Source: CAD feature listing. Evaluate the final solid. Frame: model axes, mm. A direction names the side the tool comes from. Coordinates: 2 decimals unless noted, no trailing zeros. Loops run counter-clockwise (first coordinate to the right, second up) from the corner with the lowest first, then second, coordinate; pieces in that order, holes last. Notation, with made-up numbers: M -36,48.5 L 22,48.5 A30 ccw 22,76.5 Z; hole C 38.5,43.25 d11. An arc over 180 degrees is marked long. One line per question, with ' | ' between items. Start each with the question number.
1. Access query for faces 4 (the cylindrical face through (18.28, 39.51, -28.67)), 5 (the cylindrical face through (0, 2, 41)). Directions: +Z, -Z, +X, -X, +Y, -Y. A direction counts if a zero-diameter tool reaches every point of the face in a straight line with its end or side. Return the directions, or none.
2. Section query D-D, the plane z = 38.75. Output: boundary loops of the cut face in (x, y).
3. Section query C-C, the plane x = 38.75. Output: boundary loops of the cut face in (y, z), and give its area (3 significant figures).
4. Ray query, probe 1 along X at (y, z) = (2.5, 0); probe 2 along Y at (x, z) = (-18.5, -33); probe 3 along X at (y, z) = (2.95, 38.75). Return the intervals inside material, ascending.
5. Section query B-B, the plane z = 0. Output: boundary loops of the cut face in (x, y), and give its area (3 significant figures).
6. Section query A-A, the plane x = 0. Output: boundary loops of the cut face in (y, z), and give its area (3 significant figures).
7. Mould query, pull axis X, two halves, no side actions, for faces 1 (the cylindrical face through (0.099, 2.465, -36.502)), 2 (the flat face through (-1, 0, -1)), 3 (the cylindrical face through (-33.727, 2.465, 25.861)). Classes: pulls with the +X half, pulls with the -X half, needs draft (parallel to the pull), parting line crosses it, or undercut.
8. Pin query (flat end, axial travel): P1, Ø4, axis at x = 23, z = 34, coming from the +Y side; P2, Ø1.5, axis at x = -7, y = 48.5, coming from the +Z side; P3, Ø2, axis at y = 17, z = -21.5, coming from the -X side. Return the tip coordinate at first contact, or that it passes through.
```python
from build123d import *

# Parameters (mm, degrees)
ESQUISSE1_R        = 42.5
BOSS_EXTRU_2_DEPTH = 5
D_GAGEMENT_M42_D   = 4.5
ESQUISSE12_R       = 34
BOSS_EXTRU_3_DEPTH = 70


with BuildPart() as part:
    # Esquisse1 → Boss.-Extru.2 (new body)
    with BuildSketch(Plane(origin=(0, 0, 0), x_dir=(1, 0, 0), z_dir=(0, 1, 0))):
        Circle(ESQUISSE1_R)
    extrude(amount=BOSS_EXTRU_2_DEPTH)

    # Dégagement M42 (through all)
    with Locations(Plane(origin=(0, 5, -38.75), x_dir=(0, 0, 1), z_dir=(0, 1, 0))):
        with Locations((0, 0), (38.75, -38.75), (77.5, 0), (38.75, 38.75)):
            Hole(D_GAGEMENT_M42_D / 2)

    # Esquisse12 → Boss.-Extru.3 (add)
    with BuildSketch(Plane(origin=(0, 5, 0), x_dir=(1, 0, 0), z_dir=(0, 1, 0))):
        Circle(ESQUISSE12_R)
    extrude(amount=BOSS_EXTRU_3_DEPTH)


solid = part.part
```
Taken from the geometry:
1) face 4: +Y | face 5: +Y, -Y
2) outline: M -17.46,0 L -2.25,0 L -2.25,5 L -17.46,5 Z; M 2.25,0 L 17.46,0 L 17.46,5 L 2.25,5 Z
3) outline: M 0,-17.46 L 5,-17.46 L 5,-2.25 L 0,-2.25 Z; M 0,2.25 L 5,2.25 L 5,17.46 L 0,17.46 Z | area: 152 mm^2
4) probe 1: -42.5 to -41, -36.5 to 36.5, 41 to 42.5 | probe 2: 0 to 5 | probe 3: -17.46 to -2.25, 2.25 to 17.46
5) outline: M -42.5,0 L -41,0 L -41,5 L -42.5,5 Z; M -36.5,0 L 36.5,0 L 36.5,5 L 34,5 L 34,75 L -34,75 L -34,5 L -36.5,5 Z; M 41,0 L 42.5,0 L 42.5,5 L 41,5 Z | area: 5,140 mm^2
6) outline: M 0,-42.5 L 5,-42.5 L 5,-41 L 0,-41 Z; M 0,-36.5 L 5,-36.5 L 5,-34 L 75,-34 L 75,34 L 5,34 L 5,36.5 L 0,36.5 Z; M 0,41 L 5,41 L 5,42.5 L 0,42.5 Z | area: 5,140 mm^2
7) face 1: undercut | face 2: needs draft | face 3: parting line crosses it
8) P1: y = 5 | P2: z = 33.42 | P3: x = -27.12
